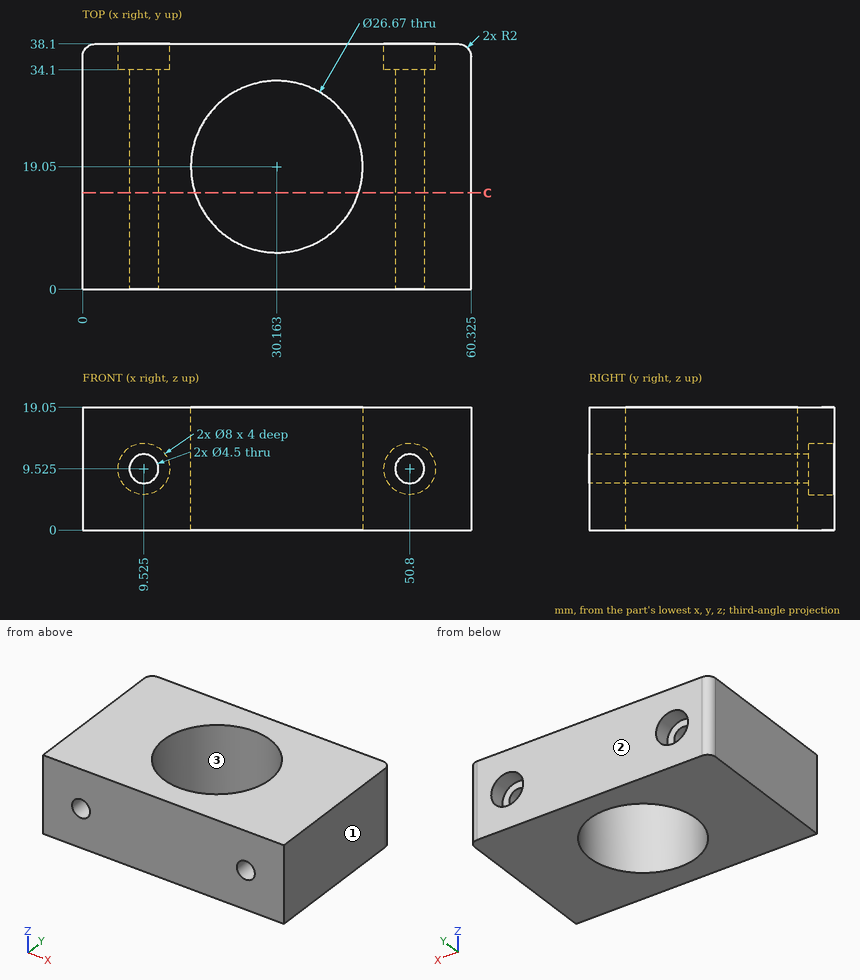
Geometry check sheet. Reference: drawing and pictorial views, mm from the part's lowest x, y, z. Give positions to 0.01 mm unless a question says otherwise; leave off trailing zeros. Answer as CSV lines item,"result". Start each with the question number.
Item 1: Section check C-C, the plane y = 15. State how many separate pieces and enclosed holes the cut face has, plus the area to 3 significant figures.
Item 2: Gauge pin test, flat end, axial feed: pin 1 (5 mm diameter, centred on x = 9.525, z = 9.525, fed in from +Y). Record the tip position at first contact, or that the pin passes through.
Item 3: Material ranges on L1, parallel to X at y = 19.5, z = 1.75 (1 decimal); L2, parallel to X at y = 4, z = 11 (1 decimal); L3, parallel to X at y = 25, z = 8.5 (1 decimal), recorded low to high.
Item 4: Mould release check, pull along X, two halves, no side actions. Record for the marked faces 1, 2 and 3: released by +X, released by -X, zero draft, split by the parting line, or undercut.
Filled in:
1,separate pieces,"2"
1,enclosed holes,"2"
1,area,"633 mm^2"
2,pin 1,"y = 34.1"
3,L1,"0 to 16.8, 43.5 to 60.3"
3,L2,"0 to 7.8, 11.2 to 49.1, 52.5 to 60.3"
3,L3,"0 to 7.5, 11.5 to 18.2, 42.1 to 48.8, 52.8 to 60.3"
4,face 1,"released by +X"
4,face 2,"zero draft"
4,face 3,"undercut"
